The model under review builds one solid part; all positions refer to its coordinate system, in mm. A direction names the side the tool comes from. Round coordinates to 2 decimals unless told otherwise and drop trailing zeros. Loops run counter-clockwise (first coordinate to the right, second up) from the corner with the lowest first, then second, coordinate; pieces in that order, holes last. Notation, with made-up numbers: (13, -15.5) -> (55, -15.5) arc R22 cw to (55, 12.5) -> close; hole circle Ø3 at (-22, 33). An arc over 180 degrees is marked (long way). Return JSON: item names as keys, results as strings. Group by question number.
```python
from build123d import *

# Parameters (mm, degrees)
SKETCH1_W           = 50
SKETCH1_H           = 45
BOSS_EXTRUDE1_DEPTH = 5
SKETCH2_W           = 10
SKETCH2_H           = 10
BOSS_EXTRUDE2_DEPTH = 20


with BuildPart() as part:
    # Sketch1 → Boss-Extrude1 (new body)
    with BuildSketch(Plane(origin=(0, 0, 0), x_dir=(1, 0, 0), z_dir=(0, 1, 0))):
        with Locations((0.556666279, -1.630839984)):
            Rectangle(SKETCH1_W, SKETCH1_H)
        with BuildLine():
            Line((-7.4, -15), (-7.4, -10.223338333))
            ThreePointArc((-7.4, -10.223338333), (-7.449237284, -10.031074147), (-7.584827586, -9.886142793))
            ThreePointArc((-7.584827586, -9.886142793), (0, 16.1), (7.584827586, -9.886142793))
            ThreePointArc((7.584827586, -9.886142793), (7.449237284, -10.031074147), (7.4, -10.223338333))
            Line((7.4, -10.223338333), (7.4, -15))
            ThreePointArc((7.4, -15), (7.077817459, -15.777817459), (6.3, -16.1))
            Line((6.3, -16.1), (-6.3, -16.1))
            ThreePointArc((-6.3, -16.1), (-7.077817459, -15.777817459), (-7.4, -15))
        make_face(mode=Mode.SUBTRACT)
    extrude(amount=BOSS_EXTRUDE1_DEPTH)

    # Sketch2 → Boss-Extrude2 (add)
    with BuildSketch(Plane.XZ):
        with Locations((-19.443333721, 19.130839984)):
            Rectangle(SKETCH2_W, SKETCH2_H)
        with Locations((-19.443333721, -15.869160016)):
            Rectangle(SKETCH2_W, SKETCH2_H)
        with Locations((20.556666279, -15.869160016)):
            Rectangle(SKETCH2_W, SKETCH2_H)
        with Locations((20.556666279, 19.130839984)):
            Rectangle(SKETCH2_W, SKETCH2_H)
    extrude(amount=BOSS_EXTRUDE2_DEPTH)


solid = part.part
```
1. Draft analysis for pull direction Z (two halves, no side actions). For faces 1 (the face through (20, -20, 19)), 2 (the face through (-0.51, 2.46, -16.09)), 3 (the face through (0, 1, 24.131)), state which applies: pulls with the +Z half, pulls with the -Z half, needs draft (parallel to the pull), parting line crosses it, or undercut.
2. We need section A-A, the plane z = -2. Write out the cut boundary in (x, y), then the cut area to 3 significant figures.
3. We need section C-C, the plane x = 0. Write out the cut boundary in (y, z).
4. We need section B-B, the plane y = -8.5. Write out the cut boundary in (x, z), then the cut area to 3 significant figures.
5. Wall thickness on line 1 (X direction, y = 3.25, z = 13); line 2 (X direction, y = -10, z = -16); line 3 (Z direction, x = 19, y = -3.25): over which ranges is each line inside the solid? List them lowest first.
6. We need section D-D, the plane z = 19.5. Write out the cut boundary in (x, y).
7. Tool access review of faces 4 (the face through (-7.069, 2.465, 15.786)), 5 (the face through (15.557, -10, -16)), 6 (the face through (-20, -10, 14.131)): name each direction out of +Z, -Z, +X, -X, +Y, -Y from which nothing blocks a thin tool from reaching the whole face with its end or side.
8. For P1, Ø12, axis at y = -12, z = -3.5, coming from the -X side, flat-tipped, find the tip position at first contact; note if it passes through.
Check sheet entries:
{
 "1": {"face 1": "needs draft", "face 2": "undercut", "face 3": "pulls with the +Z half"},
 "2": {"outline": "(-24.44, 0) -> (-14.1, 0) -> (-14.1, 5) -> (-24.44, 5) -> close; (14.1, 0) -> (25.56, 0) -> (25.56, 5) -> (14.1, 5) -> close", "area": "109 mm²"},
 "3": {"outline": "(0, -20.87) -> (5, -20.87) -> (5, -16.1) -> (0, -16.1) -> close; (0, 16.1) -> (5, 16.1) -> (5, 24.13) -> (0, 24.13) -> close"},
 "4": {"outline": "(-24.44, -20.87) -> (-14.44, -20.87) -> (-14.44, -10.87) -> (-24.44, -10.87) -> close; (-24.44, 14.13) -> (-14.44, 14.13) -> (-14.44, 24.13) -> (-24.44, 24.13) -> close; (15.56, -20.87) -> (25.56, -20.87) -> (25.56, -10.87) -> (15.56, -10.87) -> close; (15.56, 14.13) -> (25.56, 14.13) -> (25.56, 24.13) -> (15.56, 24.13) -> close", "area": "400 mm²"},
 "5": {"line 1": "x = -24.44 to -7.4, 7.4 to 25.56", "line 2": "x = -24.44 to -14.44, 15.56 to 25.56", "line 3": "z = -20.87 to -10.87, 14.13 to 24.13"},
 "6": {"outline": "(-24.44, -20) -> (-14.44, -20) -> (-14.44, 0) -> (15.56, 0) -> (15.56, -20) -> (25.56, -20) -> (25.56, 5) -> (-24.44, 5) -> close"},
 "7": {"face 4": "+Y, -Y", "face 5": "+Z, -Z, -Y", "face 6": "+X, -X, -Y"},
 "8": {"P1": "passes through"}
}
